The listing builds one solid part. Answer for the finished solid, in the listing's coordinates (mm). Give positions to 0.01 mm unless a question says otherwise; leave off trailing zeros. Order: outer loops, then holes, each group sorted by start corner. A loop starts at its lowest first (then second) coordinate and runs counter-clockwise, first axis right, second up. Notation, with made-up numbers: (-23.5, 77.25) -> (20.5, 77.25) arc R34 cw to (20.5, 108.25) -> close; hole circle Ø1 at (-27, 62). An arc over 180 degrees is marked (long way). Answer as a JSON object with one key per item and string values. Group by question number.
```python
from build123d import *

# Parameters (mm, degrees)
F0_R     = 14.28115
F1_DEPTH = 6
F2_R     = 14.2875
F2_R_2   = 2.5527
F3_DEPTH = 25.4
F5_D     = 5.1054


with BuildPart() as f1:
    # F0 (on Front) → F1 (new body)
    with BuildSketch(Plane.XZ):
        Polygon((203.2, -152.4), (203.2, 152.4), (203.2, 203.2), (-101.6, 203.2), (-101.6, 152.4), (152.4, 152.4), (152.4, -152.4), (-101.6, -152.4), (-101.6, -203.2), (203.2, -203.2), align=None)
        with Locations((-76.2, -177.8)):
            Circle(F0_R, mode=Mode.SUBTRACT)
        with Locations((-76.2, 177.8)):
            Circle(F0_R, mode=Mode.SUBTRACT)
    extrude(amount=F1_DEPTH)

    # F2 (on face) → F3 (cut)
    with BuildSketch(Plane.XZ.offset(6)):
        with Locations((152.4, 177.8)):
            Circle(F2_R)
        with Locations((169.926, 195.326)):
            Circle(F2_R_2)
        with Locations((169.926, 160.274)):
            Circle(F2_R_2)
        with Locations((134.874, 160.274)):
            Circle(F2_R_2)
        with Locations((134.874, 195.326)):
            Circle(F2_R_2)
        with Locations((134.874, -195.326)):
            Circle(F2_R_2)
        with Locations((134.874, -160.274)):
            Circle(F2_R_2)
        with Locations((169.926, -160.274)):
            Circle(F2_R_2)
        with Locations((152.4, -177.8)):
            Circle(F2_R)
        with Locations((169.926, -195.326)):
            Circle(F2_R_2)
    extrude(amount=-F3_DEPTH, mode=Mode.SUBTRACT)

    # F5 (through all)
    with Locations(Plane.XZ.offset(6)):
        with Locations((114.3, 190.5), (114.3, 165.100002), (88.9, 165.100002), (-38.1, 190.5), (12.7, 190.5), (63.5, 165.100002), (88.9, 190.5), (63.5, 190.5), (-38.1, 165.100002), (38.1, 165.100002), (38.1, 190.5), (-12.7, 190.5), (12.7, 165.100002), (-12.7, 165.100002), (190.5, 165.100002), (190.5, 190.5), (114.3, -165.100002), (-38.1, -190.5), (-12.7, -165.100002), (38.1, -165.100002), (-38.1, -165.100002), (-12.7, -190.5), (88.9, -190.5), (12.7, -190.5), (63.5, -165.100002), (12.7, -165.100002), (114.3, -190.5), (88.9, -165.100002), (38.1, -190.5), (63.5, -190.5), (190.5, -165.100002), (190.5, -190.5), (190.5, 139.700004), (165.100002, 139.700004), (190.5, 114.300007), (165.100002, 114.300007), (190.5, 88.900009), (165.100002, 88.900009), (190.5, 63.500011), (165.100002, 63.500011), (190.5, 38.100013), (165.100002, 38.100013), (190.5, 12.700015), (165.100002, 12.700015), (190.5, -12.699983), (165.100002, -12.699983), (190.5, -38.09998), (165.100002, -38.09998), (190.5, -63.499978), (165.100002, -63.499978), (190.5, -88.899976), (165.100002, -88.899976), (190.5, -114.299974), (165.100002, -114.299974), (190.5, -139.699972), (165.100002, -139.699972)):
            Hole(F5_D / 2)


solid = f1.part
```
(1) A cutting plane is placed at A-A (z = 177.8). Determine the outline of the cut face in (x, y), and give its area (3 significant figures).
(2) A cutting plane is placed at C-C (z = -29). Determine the outline of the cut face in (x, y), and give its area (3 significant figures).
(3) Find the intervals of material crossed by line 1 along Z through (x, y) = (63, -3.1); line 2 along X through (y, z) = (-3.2, 88.5); line 3 along X through (y, z) = (-5, 38), in increasing order. Write a range as [from, to].
(4) For a pull along Z with two mould halves and no side action, classify faces 1 (the flat face through (163, 0, 1)), 2 (the cylindrical face through (-87.533, -2.958, 169.11)) as +Z half, -Z half, draft (parallel to the pull), parting line (faces both ways), or undercut.
(5) Flat-ended cylindrical pins translate along their axes: pin 1 Ø3 at (x, z) = (134.874, -195.326) entering from +Y; pin 2 Ø6.5 at (x, z) = (190.5, -63.5) entering from -Y. Find the tip coordinate at first contact, or state that the pin passes through.
(6) A cutting plane is placed at D-D (y = -2.3). State how many separate pieces and enclosed holes the cut face has, and give its area (3 significant figures).
(7) A cutting plane is placed at B-B (x = -76.2). Determine the outline of the cut face in (y, z).
Check sheet entries:
{
 "1": {"outline": "(-101.6, -6) -> (-90.48, -6) -> (-90.48, 0) -> (-101.6, 0) -> close; (-61.92, -6) -> (138.11, -6) -> (138.11, 0) -> (-61.92, 0) -> close; (166.69, -6) -> (203.2, -6) -> (203.2, 0) -> (166.69, 0) -> close", "area": "1,490 mm2"},
 "2": {"outline": "(152.4, -6) -> (203.2, -6) -> (203.2, 0) -> (152.4, 0) -> close", "area": "305 mm2"},
 "3": {"line 1": "z = [-203.2, -193], [-188, -167.6], [-162.6, -152.4], [152.4, 162.6], [167.6, 188], [193, 203.2]", "line 2": "x = [152.4, 162.58], [167.62, 187.98], [193.02, 203.2]", "line 3": "x = [152.4, 162.55], [167.65, 187.95], [193.05, 203.2]"},
 "4": {"face 1": "draft", "face 2": "undercut"},
 "5": {"pin 1": "passes through", "pin 2": "stops at y = -6"},
 "6": {"separate pieces": "1", "enclosed holes": "68", "area": "42,600 mm2"},
 "7": {"outline": "(-6, -203.2) -> (0, -203.2) -> (0, -192.08) -> (-6, -192.08) -> close; (-6, -163.52) -> (0, -163.52) -> (0, -152.4) -> (-6, -152.4) -> close; (-6, 152.4) -> (0, 152.4) -> (0, 163.52) -> (-6, 163.52) -> close; (-6, 192.08) -> (0, 192.08) -> (0, 203.2) -> (-6, 203.2) -> close"}
}
